The listing builds one solid part. Answer for the finished solid, in the listing's coordinates (mm). A direction names the side the tool comes from. Coordinates: 2 decimals unless noted, no trailing zeros. Order: outer loops, then holes, each group sorted by start corner. A loop starts at its lowest first (then second) coordinate and runs counter-clockwise, first axis right, second up. Notation, with made-up numbers: (19, -2.75) - (25, -2.75) arc R22 cw to (25, 12.25) - close; hole circle Ø2 at (56.5, 60). An arc over 180 degrees is marked (long way). Use a Markdown table: item, result. Add a question column.
Item 1: Find the intervals of material crossed by line 1 along Y through (x, z) = (0, 0.45); line 2 along Y through (x, z) = (0, 0.8); line 3 along Z through (x, y) = (-0.25, 3), in increasing order.
Item 2: The part is cut by section A-A, the plane x = 0. Give the vertices of the cut face in (y, z).
Item 3: Flat-ended cylindrical pins translate along their axes: P1, Ø1, axis at y = -3, z = 4, coming from the +X side; P2, Ø1, axis at y = 0.5, z = 6, coming from the +X side; P3, Ø1, axis at x = -2, z = 3, coming from the -Y side; P4, Ø2.5, axis at x = 0, y = 0, coming from the -Z side. Find the tip coordinate at first contact, or state that the pin passes through.
Item 4: The part is cut by section D-D, the plane x = -4.5. Give the vertices of the cut face in (y, z), then the cut area to 3 significant figures.
Item 5: For faces 1 (the flat face through (1, 2, 7.25)), 2 (the cylindrical face through (-2.947, 0.13, 4.208)), 3 (the flat face through (-2, -1, 0.6)), determine the directions among +Z, -Z, +X, -X, +Y, -Y from which every point of the face is accessible in a straight line to the end or side of a thin tool.
Item 6: The mould has two halves that part along X. Classify faces 4 (the cylindrical face through (-1.08, -4.88, 0.62)), 5 (the cylindrical face through (3.047, 0.134, 0.296)), 6 (the flat face through (2.2, -2.2, 1.25)): released by +X, released by -X, zero draft, split by the parting line, or undercut.
Item 7: The part is cut by section C-C, the plane y = 2.25. Give the vertices of the cut face in (x, z).
from build123d import *

# Parameters (mm, degrees)
SKETCH1_R           = 5
BOSS_EXTRUDE1_DEPTH = 1.25
SKETCH2_R           = 2.95
SKETCH2_R_2         = 2.05
BOSS_EXTRUDE2_DEPTH = 6
SKETCH4_R           = 2.05
CUT_EXTRUDE3_DEPTH  = 2.25
SKETCH5_R           = 3.05
CUT_EXTRUDE4_DEPTH  = 0.6


with BuildPart() as part:
    # Sketch1 → Boss-Extrude1 (new body)
    with BuildSketch(Plane.XY):
        Circle(SKETCH1_R)
    extrude(amount=BOSS_EXTRUDE1_DEPTH)

    # Sketch2 → Boss-Extrude2 (add)
    with BuildSketch(Plane.XY.offset(1.25)):
        Circle(SKETCH2_R)
        Circle(SKETCH2_R_2, mode=Mode.SUBTRACT)
    extrude(amount=BOSS_EXTRUDE2_DEPTH)

    # Sketch4 → Cut-Extrude3 (cut, through all)
    with BuildSketch(Plane.XY.offset(1.25)):
        Circle(SKETCH4_R)
    extrude(amount=-CUT_EXTRUDE3_DEPTH, mode=Mode.SUBTRACT)

    # Sketch5 → Cut-Extrude4 (cut)
    with BuildSketch(Plane(origin=(0, 0, 0), x_dir=(-1, 0, 0), z_dir=(0, 0, -1))):
        Circle(SKETCH5_R)
    extrude(amount=-CUT_EXTRUDE4_DEPTH, mode=Mode.SUBTRACT)


solid = part.part
Solution:
| question | item | result |
|---|---|---|
| 1 | line 1 | y = -5 to -3.05, 3.05 to 5 |
| 1 | line 2 | y = -5 to -2.05, 2.05 to 5 |
| 1 | line 3 | z = 0.6 to 1.25 |
| 2 | outline | (-5, 0) - (-3.05, 0) - (-3.05, 0.6) - (-2.05, 0.6) - (-2.05, 7.25) - (-2.95, 7.25) - (-2.95, 1.25) - (-5, 1.25) - close; (2.05, 0.6) - (3.05, 0.6) - (3.05, 0) - (5, 0) - (5, 1.25) - (2.95, 1.25) - (2.95, 7.25) - (2.05, 7.25) - close |
| 3 | P1 | stops at x = 1.57 |
| 3 | P2 | stops at x = 2.95 |
| 3 | P3 | stops at y = -2.54 |
| 3 | P4 | passes through |
| 4 | outline | (-2.18, 0) - (2.18, 0) - (2.18, 1.25) - (-2.18, 1.25) - close |
| 4 | area | 5.45 mm2 |
| 5 | face 1 | +Z, +X, -X, +Y, -Y |
| 5 | face 2 | +Z |
| 5 | face 3 | -Z |
| 6 | face 4 | split by the parting line |
| 6 | face 5 | undercut |
| 6 | face 6 | zero draft |
| 7 | outline | (-4.47, 0) - (-2.06, 0) - (-2.06, 0.6) - (2.06, 0.6) - (2.06, 0) - (4.47, 0) - (4.47, 1.25) - (1.91, 1.25) - (1.91, 7.25) - (-1.91, 7.25) - (-1.91, 1.25) - (-4.47, 1.25) - close |
